Autodesk Inventor part; units mm, degrees
ref_plane "YZ Plane" through (0, 0, 0) normal (1, 0, 0) x (0, 1, 0)
ref_plane "XZ Plane" through (0, 0, 0) normal (0, 1, 0) x (-1, 0, 0)
ref_plane "XY Plane" through (0, 0, 0) normal (0, 0, 1) x (1, 0, 0)
ref_plane "Work Plane1" through (0, 0, -3.175) normal (0, 0, -1) x (-1, 0, 0)
sketch "Sketch1" plane through (0, 0, -3.175) normal (0, 0, -1) x (-1, 0, 0)
  circle A0 centre (171.45, -37.338) radius 2.667
  circle A1 centre (184.15, -11.938) radius 2.667
  circle A2 centre (577.85, 750.062) radius 2.667 construction
  circle A3 centre (565.15, 724.662) radius 2.667 construction
  line L0 (0, 763.524) -> (736.6, 763.524)
  line L1 (736.6, -50.8) -> (0, -50.8)
  line L2 (154.0806, -50.8) -> (541.7292, 763.524)
  line L3 (582.5194, 763.524) -> (194.8708, -50.8)
  line L4 (194.8708, -50.8) -> (154.0806, -50.8)
  line L5 (541.7292, 763.524) -> (582.5194, 763.524)
  line L6 (487.8257, 564.3774) -> (487.8257, 502.6234) construction
  line L7 (594.2009, 565.5044) -> (496.0553, 565.5044) construction
  line L8 (488.8257, 565.3774) -> (496.0553, 565.3774) construction
  line L9 (248.7743, 148.3466) -> (248.7743, 210.1006) construction
  line L10 (247.7743, 147.3466) -> (240.5447, 147.3466) construction
  line L11 (142.3991, 147.2196) -> (240.5447, 147.2196) construction
  arc A4 (247.7743, 147.3466) -> (248.7743, 148.3466) centre (247.7743, 148.3466) ccw construction
  arc A5 (488.8257, 565.3774) -> (487.8257, 564.3774) centre (488.8257, 564.3774) ccw construction
  line L12 (622.3, 759.587) -> (622.3, 435.737) construction
  line L13 (114.3, -46.863) -> (114.3, 276.987) construction
  circle A6 centre (565.15, 750.062) radius 2.667
  circle A7 centre (552.45, 724.662) radius 2.667
  point P0 (0, 0)
  dimension "d0" = 36.83
  dimension "d1" = 39.7806
extrude "Extrusion1" add sketch "Sketch1" against normal blind 19.2659
properties part number "FR-RL Wood Brace"
Geometry check sheet. Reference: the model listing, model coordinates, mm. Give positions to 0.01 mm unless a question says otherwise; leave off trailing zeros. Order: outer loops, then holes, each group sorted by start corner. A loop starts at its lowest first (then second) coordinate and runs counter-clockwise, first axis right, second up.
1. Draft check along Y on faces 1 (the face through (-175, -50.8, 6)), 2 (the face through (-345.19, 350.66, 6.32)), 3 (the face through (-367, 358, 16.091)). Enter one of: pulls with the +Y half, pulls with the -Y half, needs draft (parallel to the pull), parting line crosses it, or undercut.
Completed:
face 1: pulls with the -Y half
face 2: pulls with the +Y half
face 3: needs draft
2. Depth check by flat-ended pin: pin 1 (8.5 mm diameter, centred on x = -184.15, y = -11.938, fed in from +Z); pin 2 (4 mm diameter, centred on x = -459.5, z = 12, fed in from +Y); pin 3 (4 mm diameter, centred on y = 586, z = 8, fed in from -X); pin 4 (5 mm diameter, centred on y = 216.5, z = 13, fed in from -X). Enter the tip coordinate at first touch or a pass-through.
Completed:
pin 1: stops at z = 16.09
pin 2: stops at y = 594.99
pin 3: stops at x = -498.96
pin 4: stops at x = -323.31
3. Sectioned sample at B-B (y = 526.5). Record the boundary of the cut face in (x, z) (3 decimals), then the cut area to 3 significant figures.
Completed:
outline: (-469.687, -3.175) - (-428.897, -3.175) - (-428.897, 16.091) - (-469.687, 16.091) - close
area: 786 mm2
4. Scan lines: line 1 (Y direction, x = -552.45, z = 6.5) (3 decimals); line 2 (Y direction, x = -550.5, z = 14.5); line 3 (Y direction, x = -216.5, z = 8.25). Record each from-to range of solid material in increasing order.
Completed:
line 1: y = 700.358 to 721.995, 727.329 to 763.524
line 2: y = 696.26 to 722.84, 726.48 to 763.52
line 3: y = -5.36 to 80.32
5. Sectioned sample at A-A (z = 5.5). Record the boundary of the cut face in (x, y), then the cut area to 3 significant figures.
Completed:
outline: (-582.52, 763.52) - (-194.87, -50.8) - (-154.08, -50.8) - (-541.73, 763.52) - close; hole circle Ø5.33 at (-565.15, 750.06); hole circle Ø5.33 at (-552.45, 724.66); hole circle Ø5.33 at (-184.15, -11.94); hole circle Ø5.33 at (-171.45, -37.34)
area: 33,100 mm2
6. Sectioned sample at C-C (x = -444). Record the boundary of the cut face in (y, z) (3 decimals), then the cut area to 3 significant figures.
Completed:
outline: (472.54, -3.175) - (558.227, -3.175) - (558.227, 16.091) - (472.54, 16.091) - close
area: 1,650 mm2
